Solid Edge part; units mm, degrees
sketch "Sketch1" plane through (0, 0, 0) normal (0, -1, 0) x (1, 0, 0)
  line L0 (0, 0) -> (3.75, 0)
  line L1 (3.75, 0) -> (2, -1.75)
  line L2 (2, -1.75) -> (2, -41.75)
  line L3 (2, -41.75) -> (0, -41.75)
  dimension "D1" = 2
revolve "RevolvedProtrusion1" add sketch "Sketch1" angle 360 about axis through (0, 0, -21.75) along (0, 0, 1)
chamfer "end_chamfer" distance 0.5 angle 45 1 edges at (-2, 0, -41.75)
sketch "Sketch2" plane through (0, 0, 0) normal (0, 0, 1) x (0, 1, 0)
  line L0 (0.5, -0.5) -> (2, -0.5)
  line L1 (2, -0.5) -> (2, 0.5)
  line L2 (2, 0.5) -> (0.5, 0.5)
  line L3 (0.5, 2) -> (0.5, 0.5)
  line L4 (-0.5, 2) -> (0.5, 2)
  line L5 (-0.5, 0.5) -> (-0.5, 2)
  line L6 (-0.5, 0.5) -> (-2, 0.5)
  line L7 (-2, 0.5) -> (-2, -0.5)
  line L8 (-2, -0.5) -> (-0.5, -0.5)
  line L9 (-0.5, -2) -> (-0.5, -0.5)
  line L10 (0.5, -2) -> (-0.5, -2)
  line L11 (0.5, -0.5) -> (0.5, -2)
  dimension "D1" = 0.5
extrude "x_slot" cut sketch "Sketch2" against normal blind 1.2
cosmetic_thread "Thread1"
properties part number "STD-DIN965-M4x40" material "Stainless steel"
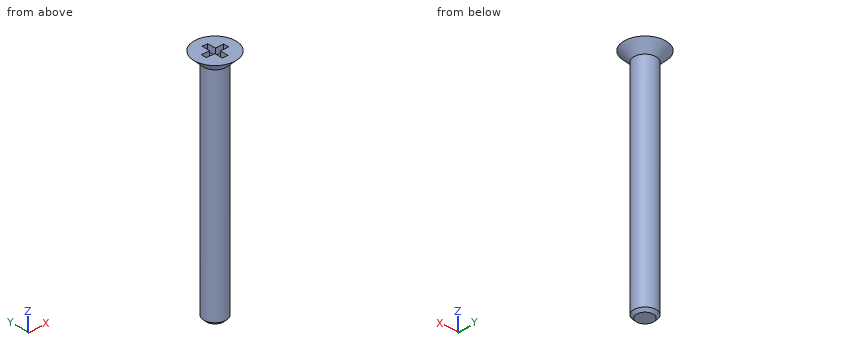
CAD build for the part. Positions are in the model's coordinates, mm. Coordinates: 2 decimals unless noted, no trailing zeros. Write each loop counter-clockwise with the first axis right and the second up, starting at its lowest first coordinate (ties: lowest second). Pieces come first, ordered by that corner, then holes.
(1) Cut at A-A, the plane x = 0. List the corners of the cut face in (y, z), and give its area (3 significant figures).
(2) Drill centre lines: probe 1 along Z at (x, y) = (-2.25, 0); probe 2 along Y at (x, z) = (-1.75, -39.5); probe 3 along Y at (x, z) = (0.75, -9). Where is each one in solid material? Low to high.
(3) Flat gauge pins, fed straight in: pin 1 (1.1 mm diameter, centred on x = 0, z = -1, fed in from -Y); pin 2 (1.5 mm diameter, centred on x = -2.5, z = -15, fed in from -Y); pin 3 (1 mm diameter, centred on y = -1.5, z = -0.5, fed in from -X). Where does each tip first touch, or does it go through?
(4) Cut at C-C, the plane z = -18. List the corners of the cut face in (x, y), and give its area (3 significant figures).
Geometry says:
1. outline: (-3.75, 0) - (-2, -1.75) - (-2, -41.25) - (-1.5, -41.75) - (1.5, -41.75) - (2, -41.25) - (2, -1.75) - (3.75, 0) - (2, 0) - (2, -1.2) - (-2, -1.2) - (-2, 0) - close
1. area: 165 mm2
2. probe 1: z = -1.5 to 0
2. probe 2: y = -0.97 to 0.97
2. probe 3: y = -1.85 to 1.85
3. pin 1: stops at y = -3.3
3. pin 2: stops at y = -0.97
3. pin 3: stops at x = -3.47
4. outline: circle Ø4 at (0, 0)
4. area: 12.6 mm2
